from build123d import *

# Parameters (mm, degrees)
BOSS_EXTRUDE1_DEPTH = 12.7
SKETCH2_R           = 3.556
CUT_EXTRUDE1_DEPTH  = 2.9972
SKETCH3_W           = 30.48
SKETCH3_H           = 30.48
SKETCH3_W_2         = 25.4
SKETCH3_H_2         = 25.4
BOSS_EXTRUDE2_DEPTH = 63.5
CUT_EXTRUDE2_REACH  = 114.231
SKETCH4_R           = 2.413
CUT_EXTRUDE3_DEPTH  = 12.7


with BuildPart() as part:
    # Sketch1 → Boss-Extrude1 (new body)
    with BuildSketch(Plane(origin=(0, 0, 0), x_dir=(1, 0, 0), z_dir=(0, 1, 0))):
        Polygon((-87.376, 0), (0, 0), (0, -63.5), (-87.376, -20.644), align=None)
    extrude(amount=BOSS_EXTRUDE1_DEPTH)

    # Sketch2 → Cut-Extrude1 (cut)
    with BuildSketch(Plane.ZY.offset(87.376)):
        with Locations((14.548, 6.35)):
            Circle(SKETCH2_R)
    extrude(amount=-CUT_EXTRUDE1_DEPTH, mode=Mode.SUBTRACT)

    # Sketch3 → Boss-Extrude2 (add)
    with BuildSketch(Plane(origin=(0, 0, 0), x_dir=(-1, 0, 0), z_dir=(0, 0, -1))):
        with Locations((-12.7, 6.35)):
            Rectangle(SKETCH3_W, SKETCH3_H)
        with Locations((-12.7, 6.35)):
            Rectangle(SKETCH3_W_2, SKETCH3_H_2, mode=Mode.SUBTRACT)
    extrude(amount=-BOSS_EXTRUDE2_DEPTH)

    # Cut-Extrude2: up to this face of the body (flat: up to its plane)
    cut_extrude2_end = Plane(part.part.faces().sort_by_distance((12.7, -8.89, 31.75))[0])
    # Sketch4 → Cut-Extrude2 (cut, up to the picked face)
    with BuildSketch(Plane(origin=(0, 21.59, 0), x_dir=(1, 0, 0), z_dir=(0, 1, 0)), mode=Mode.PRIVATE) as cut_extrude2_sk1:
        with Locations(Location((12.7, -15.875, 0), (0, 0, 270))):
            Circle(SKETCH4_R)
    cut_extrude2_tool1 = split(extrude(cut_extrude2_sk1.sketch, amount=-CUT_EXTRUDE2_REACH, mode=Mode.PRIVATE), bisect_by=cut_extrude2_end, keep=Keep.BOTH, mode=Mode.PRIVATE)
    # Sketch4 → Cut-Extrude2 (cut, up to the picked face)
    with BuildSketch(Plane(origin=(0, 21.59, 0), x_dir=(1, 0, 0), z_dir=(0, 1, 0)), mode=Mode.PRIVATE) as cut_extrude2_sk2:
        with Locations(Location((12.7, -47.625, 0), (0, 0, 270))):
            Circle(SKETCH4_R)
    cut_extrude2_tool2 = split(extrude(cut_extrude2_sk2.sketch, amount=-CUT_EXTRUDE2_REACH, mode=Mode.PRIVATE), bisect_by=cut_extrude2_end, keep=Keep.BOTH, mode=Mode.PRIVATE)
    add(cut_extrude2_tool1.solids().sort_by(Axis((12.7, 21.59, 15.875), (0, -1, 0)))[0], mode=Mode.SUBTRACT)
    add(cut_extrude2_tool2.solids().sort_by(Axis((12.7, 21.59, 47.625), (0, -1, 0)))[0], mode=Mode.SUBTRACT)

    # Sketch8 → Cut-Extrude3 (cut)
    with BuildSketch(Plane(origin=(0, 12.7, 0), x_dir=(1, 0, 0), z_dir=(0, 1, 0))):
        Polygon((-87.376, -8.452), (-2.54, 0), (-87.376, 0), align=None)
    extrude(amount=-CUT_EXTRUDE3_DEPTH, mode=Mode.SUBTRACT)


solid = part.part
Geometry check sheet. Reference: the model listing, model coordinates, mm. A direction names the side the tool comes from. Coordinates: 2 decimals unless noted, no trailing zeros. Write each loop counter-clockwise with the first axis right and the second up, starting at its lowest first coordinate (ties: lowest second). Pieces come first, ordered by that corner, then holes. Notation, with made-up numbers: (65, 37.25) -> (99, 37.25) arc R28 cw to (99, 68.25) -> close; hole circle Ø8 at (-7, 59.25). An arc over 180 degrees is marked (long way). One line per question, with ' | ' between items.
1. Cross-section at B-B on y = 6.35. Record the cut outline in (x, z).
Answers:
outline: (-87.38, 8.45) -> (-2.54, 0) -> (0, 0) -> (0, 63.5) -> (-2.54, 63.5) -> (-2.54, 62.25) -> (-87.38, 20.64) -> (-87.38, 18.1) -> (-84.38, 18.1) -> (-84.38, 10.99) -> (-87.38, 10.99) -> close; (25.4, 0) -> (27.94, 0) -> (27.94, 63.5) -> (25.4, 63.5) -> close
2. Thickness scan on probe 1 along X at (y, z) = (12, 15.5); probe 2 along X at (y, z) = (14, 28); probe 3 along Y at (x, z) = (2.5, 8.5). Record the ranges inside material, lowest first. Write a range as from..to.
Answers:
probe 1: x = -87.38..0, 25.4..27.94 | probe 2: x = -2.54..0, 25.4..27.94 | probe 3: y = -8.89..-6.35, 19.05..21.59
3. Cross-section at D-D on z = 60. Record the cut outline in (x, y).
Answers:
outline: (-7.14, 0) -> (-2.54, 0) -> (-2.54, -8.89) -> (27.94, -8.89) -> (27.94, 21.59) -> (-2.54, 21.59) -> (-2.54, 12.7) -> (-7.14, 12.7) -> close; hole (0, -6.35) -> (25.4, -6.35) -> (25.4, 19.05) -> (0, 19.05) -> close
4. Depth check by flat-ended pin: pin 1 Ø2 at (x, y) = (-34, 8) entering from -Z; pin 2 Ø2 at (y, z) = (5.5, 13) entering from -X; pin 3 Ø4 at (x, y) = (-50, 3.5) entering from +Z. Enter the tip coordinate at first touch or a pass-through.
Answers:
pin 1: stops at z = 3.03 | pin 2: stops at x = -84.38 | pin 3: stops at z = 39.96
5. Draft check along Z on faces 6 (the flat face through (-35, 0, 24)), 7 (the flat face through (-84.379, 6, 14)), 8 (the flat face through (-1, 7, 0)). Enter one of: +Z half, -Z half, draft (parallel to the pull), parting line (faces both ways), or undercut.
Answers:
face 6: draft | face 7: undercut | face 8: -Z half
6. Set-up check for faces 1 (the flat face through (13, 21.59, 31)), 2 (the cylindrical face through (-85.898, 4.988, 17.833)), 3 (the flat face through (-87.376, 3, 12)), 4 (the flat face through (-35, 12.7, 24)), 5 (the flat face through (25.4, 6, 31)): record each of +Z, -Z, +X, -X, +Y, -Y from which the full face is reachable in a straight line by a thin tool's end or side.
Answers:
face 1: +Z, -Z, +X, -X, +Y | face 2: -X | face 3: +Z, -Z, -X, +Y, -Y | face 4: +Z, -Z, -X, +Y | face 5: +Z, -Z
7. Cross-section at A-A on x = 12.7. Record the cut outline in (y, z), and give its area (3 significant figures).
Answers:
outline: (-8.89, 0) -> (-6.35, 0) -> (-6.35, 13.46) -> (-8.89, 13.46) -> close; (-8.89, 18.29) -> (-6.35, 18.29) -> (-6.35, 45.21) -> (-8.89, 45.21) -> close; (-8.89, 50.04) -> (-6.35, 50.04) -> (-6.35, 63.5) -> (-8.89, 63.5) -> close; (19.05, 0) -> (21.59, 0) -> (21.59, 13.46) -> (19.05, 13.46) -> close; (19.05, 18.29) -> (21.59, 18.29) -> (21.59, 45.21) -> (19.05, 45.21) -> close; (19.05, 50.04) -> (21.59, 50.04) -> (21.59, 63.5) -> (19.05, 63.5) -> close | area: 274 mm²
8. Cross-section at C-C on z = 15. Record the cut outline in (x, y), and give its area (3 significant figures).
Answers:
outline: (-87.38, 0) -> (-2.54, 0) -> (-2.54, -8.89) -> (10.45, -8.89) -> (10.45, -6.35) -> (0, -6.35) -> (0, 19.05) -> (10.45, 19.05) -> (10.45, 21.59) -> (-2.54, 21.59) -> (-2.54, 12.7) -> (-87.38, 12.7) -> (-87.38, 9.88) -> (-84.38, 9.88) -> (-84.38, 2.82) -> (-87.38, 2.82) -> close; (14.95, -8.89) -> (27.94, -8.89) -> (27.94, 21.59) -> (14.95, 21.59) -> (14.95, 19.05) -> (25.4, 19.05) -> (25.4, -6.35) -> (14.95, -6.35) -> close | area: 1,320 mm²
